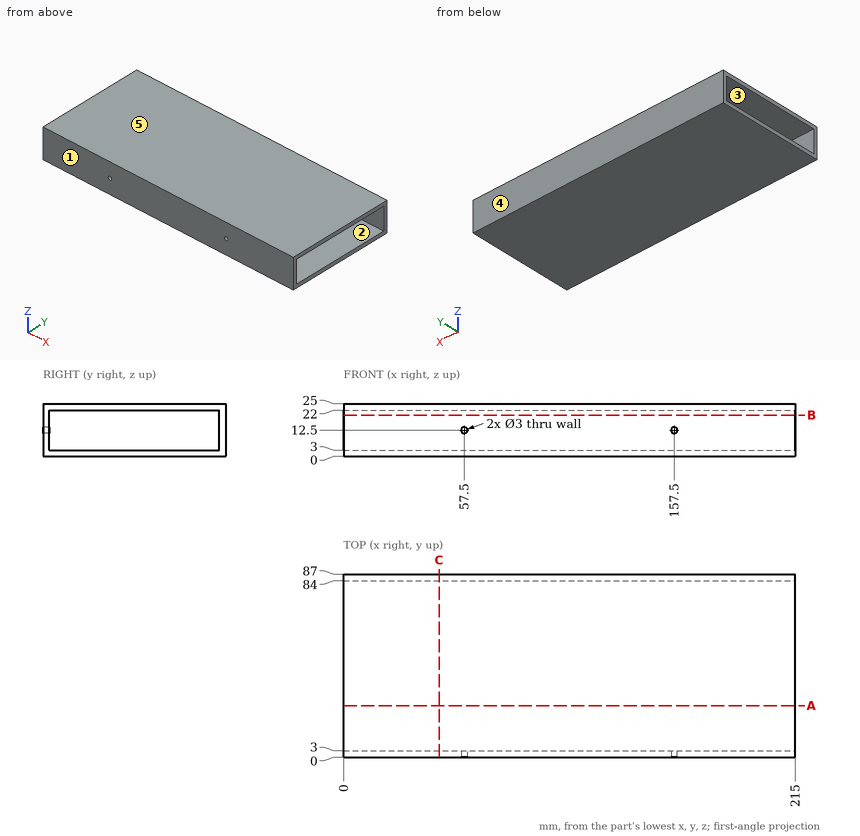
Geometry check sheet. Reference: drawing and pictorial views, mm from the part's lowest x, y, z. A direction names the side the tool comes from. Coordinates: 2 decimals unless noted, no trailing zeros. Order: outer loops, then holes, each group sorted by start corner. A loop starts at its lowest first (then second) coordinate and runs counter-clockwise, first axis right, second up. Notation, with made-up numbers: (-18, 16) -> (23, 16) arc R18 cw to (23, 32) -> close; hole circle Ø2 at (69, 21.25). An arc over 180 degrees is marked (long way). Put each result on its own line as item: value. Start each with the question number.
1) Cross-section at A-A (y = 24.5). Enter the section's corners in (x, z).
2) Cross-section at B-B (z = 19.75). Enter the section's corners in (x, y).
3) Tool access check on the marked faces 1 and 2. Record the directions out of +Z, -Z, +X, -X, +Y, -Y that give a thin tool (end or side, any length) a straight path to the whole face; none if there is none.
4) Release check for a two-part mould opening along Y. For the marked faces 3, 4 and 5 record: pulls with the +Y half, pulls with the -Y half, needs draft (parallel to the pull), parting line crosses it, or undercut.
5) Go/stop test with flat-tipped pins: pin 1 (6 mm diameter, centred on y = 75.5, z = 18, fed in from -X); pin 2 (1.8 mm diameter, centred on x = 157.5, z = 12.5, fed in from -Y). Record where each tip stops, or that it passes through.
6) Cross-section at C-C (x = 45.5). Enter the section's corners in (y, z).
7) Material ranges on L1, parallel to Y at x = 159.5, z = 21; L2, parallel to Z at x = 203, y = 10; L3, parallel to Z at x = 57.5, y = 2.2, recorded low to high.
Geometry check:
1. outline: (0, 0) -> (215, 0) -> (215, 3) -> (0, 3) -> close; (0, 22) -> (215, 22) -> (215, 25) -> (0, 25) -> close
2. outline: (0, 0) -> (215, 0) -> (215, 3) -> (0, 3) -> close; (0, 84) -> (215, 84) -> (215, 87) -> (0, 87) -> close
3. face 1: +Z, -Z, +X, -X, -Y
3. face 2: +X, -X
4. face 3: undercut
4. face 4: pulls with the +Y half
4. face 5: needs draft
5. pin 1: passes through
5. pin 2: stops at y = 84
6. outline: (0, 0) -> (87, 0) -> (87, 25) -> (0, 25) -> close; hole (3, 3) -> (84, 3) -> (84, 22) -> (3, 22) -> close
7. L1: y = 0 to 3, 84 to 87
7. L2: z = 0 to 3, 22 to 25
7. L3: z = 0 to 11, 14 to 25
